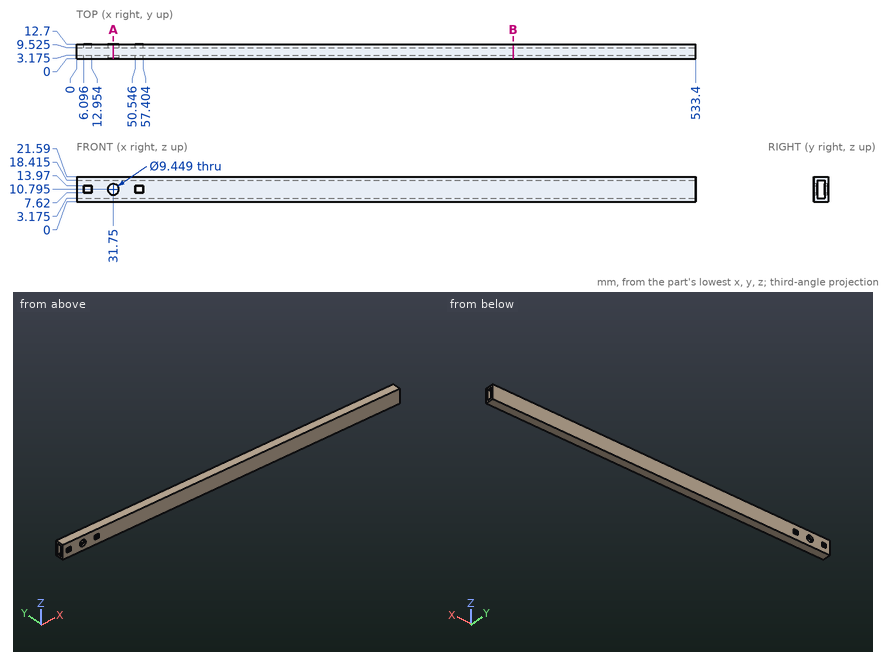
Can you work these out from the drawing? Everything is in mm from the part's minimum corner. Give positions to 0.01 mm unless a question says otherwise; leave off trailing zeros. Order: outer loops, then holes, each group sorted by start corner. A loop starts at its lowest first (then second) coordinate and runs counter-clockwise, first axis right, second up.
Item 1: If we section it at B-B, the plane x = 376: Write out the boundary of the cut face in (y, z) (3 decimals).
Item 2: If we section it at A-A, the plane x = 31.75: Write out the boundary of the cut face in (y, z) (1 decimal), plus the area to 3 significant figures.
Item 3: I'm going to push flat-ended pins straight in: pin 1 (1.6 mm diameter, centred on x = 53, y = 11.5, fed in from -Z); pin 2 (7.5 mm diameter, centred on x = 31.75, z = 10.795, fed in from +Y). Where does each tip first touch, or does it pass through?
Item 4: I need wall thicknesses on line 1 (Y direction, x = 295.5, z = 6) (3 decimals); line 2 (Z direction, x = 128, y = 4.5) (3 decimals); line 3 (X direction, y = 2.5, z = 8). Which ranges of each line are inside material? Lowest first, please.
Values:
1. outline: (0, 0) - (12.7, 0) - (12.7, 21.59) - (0, 21.59) - close; hole (3.175, 3.175) - (9.525, 3.175) - (9.525, 18.415) - (3.175, 18.415) - close
2. outline: (0, 0) - (12.7, 0) - (12.7, 6.1) - (9.5, 6.1) - (9.5, 3.2) - (3.2, 3.2) - (3.2, 6.1) - (0, 6.1) - close; (0, 15.5) - (3.2, 15.5) - (3.2, 18.4) - (9.5, 18.4) - (9.5, 15.5) - (12.7, 15.5) - (12.7, 21.6) - (0, 21.6) - close
2. area: 117 mm2
3. pin 1: stops at z = 0
3. pin 2: passes through
4. line 1: y = 0 to 3.175, 9.525 to 12.7
4. line 2: z = 0 to 3.175, 18.415 to 21.59
4. line 3: x = 0 to 6.1, 12.95 to 27.94, 35.56 to 50.55, 57.4 to 533.4
